from build123d import *


with BuildPart() as part:
    # Sketch1 → Revolve1 (revolve)
    with BuildSketch(Plane.XY):
        with BuildLine():
            Line((0, 0), (1, 0))
            Line((1, 0), (1, 39.6))
            ThreePointArc((1, 39.6), (1.117157288, 39.882842712), (1.4, 40))
            Line((1.4, 40), (2.5, 40))
            Line((2.5, 40), (2.5, 51))
            ThreePointArc((2.5, 51), (2.207106781, 51.707106781), (1.5, 52))
            Line((1.5, 52), (0, 52))
            Line((0, 52), (0, 0))
        make_face()
    revolve(axis=Axis((0, 52, 0), (0, -1, 0)))


solid = part.part
CAD build for the part. Positions are in the model's coordinates, mm. A direction names the side the tool comes from. Round coordinates to 2 decimals unless told otherwise and drop trailing zeros. Write each loop counter-clockwise with the first axis right and the second up, starting at its lowest first coordinate (ties: lowest second). Pieces come first, ordered by that corner, then holes.
(1) 3-axis set-ups, long thin cutter, end or side, ignore diameter. For faces 1 (the face through (0, 20, -1)), 2 (the face through (0, 0, 0)): which of +Z, -Z, +X, -X, +Y, -Y reach the whole face in a straight line?
(2) Slice it at C-C, the plane y = 4.5. Write the cut outline in (x, z).
(3) Probe line 1 along Z through (x, y) = (0.1, 25.5); line 2 along Y through (x, z) = (1.25, 1). List the from-to ranges inside material, lowest first.
(4) Slice it at A-A, the plane x = 0. Write the cut outline in (y, z).
(5) Drop flat-ended pins along their axis: P1, Ø1.5, axis at x = -1, z = -0.5, coming from the -Y side; P2, Ø3, axis at x = -1.5, y = 34, coming from the +Z side; P3, Ø1.5, axis at x = -1.5, y = 35, coming from the -Z side; P4, Ø2, axis at x = -1.5, y = 39.5, coming from the -Z side. Give the stop position or say it passes through.
(6) Slice it at B-B, the plane z = 0. Write the cut outline in (x, y), and give its area (3 significant figures).
(7) Slice it at D-D, the plane y = 47. Write the cut outline in (x, z).
From the geometry:
1. face 1: -Y
1. face 2: +Z, -Z, +X, -X, -Y
2. outline: circle Ø2 at (0, 0)
3. line 1: z = -0.99 to 0.99
3. line 2: y = 40 to 51.99
4. outline: (0, -1) - (39.6, -1) arc R0.4 cw to (40, -1.4) - (40, -2.5) - (51, -2.5) arc R1 ccw to (52, -1.5) - (52, 1.5) arc R1 ccw to (51, 2.5) - (40, 2.5) - (40, 1.4) arc R0.4 cw to (39.6, 1) - (0, 1) - close
5. P1: stops at y = 0
5. P2: stops at z = 1
5. P3: stops at z = -0.66
5. P4: stops at z = -2.42
6. outline: (-2.5, 40) - (-1.4, 40) arc R0.4 cw to (-1, 39.6) - (-1, 0) - (1, 0) - (1, 39.6) arc R0.4 cw to (1.4, 40) - (2.5, 40) - (2.5, 51) arc R1 ccw to (1.5, 52) - (-1.5, 52) arc R1 ccw to (-2.5, 51) - close
6. area: 140 mm2
7. outline: circle Ø5 at (0, 0)
